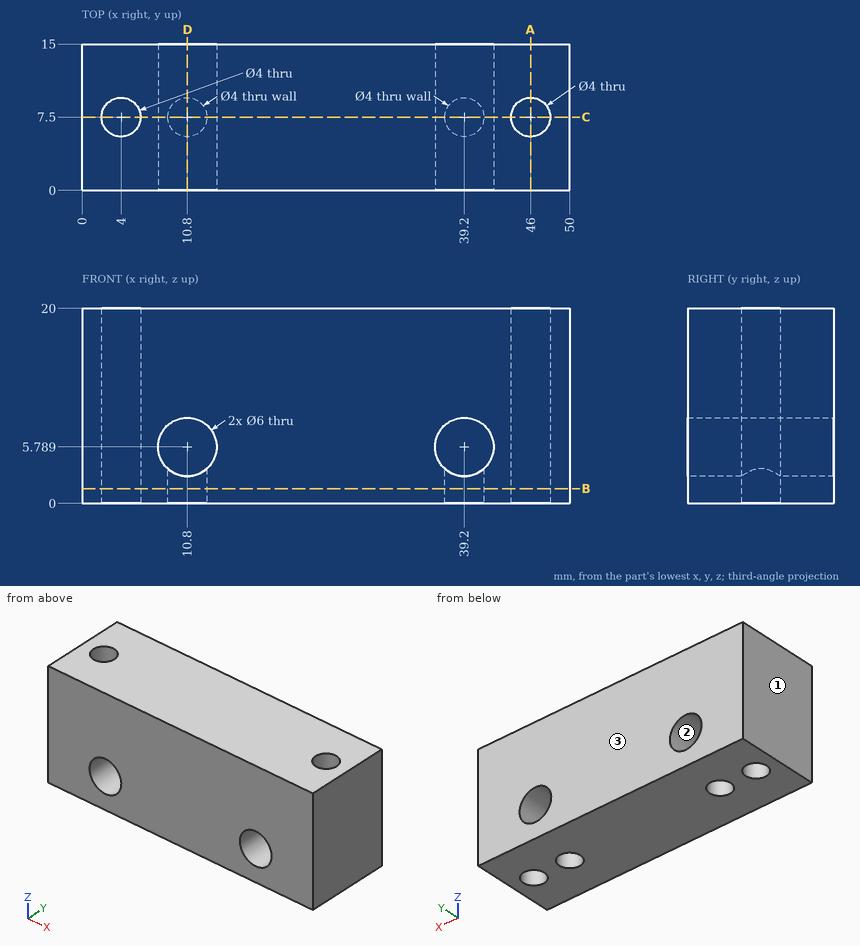
Print and shaded views of the part. All mm, measured from the part's lowest x, y and z. Round coordinates to 2 decimals unless told otherwise and drop trailing zeros. Write each loop counter-clockwise with the first axis right and the second up, starting at its lowest first coordinate (ties: lowest second). Pieces come first, ordered by that corner, then holes.
Item 1: Cut at A-A, the plane x = 46. Give the cut face in (y, z).
Results:
outline: (0, 0) - (5.5, 0) - (5.5, 20) - (0, 20) - close; (9.5, 0) - (15, 0) - (15, 20) - (9.5, 20) - close
Item 2: Two-plate mould, pull along X, no slides. Class the marked faces 1, 2 and 3: +X half, -X half, draft (parallel to the pull), parting line (faces both ways), or undercut.
Results:
face 1: -X half
face 2: undercut
face 3: draft
Item 3: Cut at D-D, the plane x = 10.8. Give the cut face in (y, z), plus the area to 3 significant figures.
Results:
outline: (0, 0) - (5.5, 0) - (5.5, 2.79) - (0, 2.79) - close; (0, 8.79) - (15, 8.79) - (15, 20) - (0, 20) - close; (9.5, 0) - (15, 0) - (15, 2.79) - (9.5, 2.79) - close
area: 199 mm2
Item 4: Cut at C-C, the plane y = 7.5. Give the cut face in (x, z), plus the area to 3 significant figures.
Results:
outline: (0, 0) - (2, 0) - (2, 20) - (0, 20) - close; (6, 0) - (8.8, 0) - (8.8, 3.55) arc R3 cw (long way) to (12.8, 3.55) - (12.8, 0) - (37.2, 0) - (37.2, 3.55) arc R3 cw (long way) to (41.2, 3.55) - (41.2, 0) - (44, 0) - (44, 20) - (6, 20) - close; (48, 0) - (50, 0) - (50, 20) - (48, 20) - close
area: 759 mm2
Item 5: Probe L1, parallel to X at y = 13.75, z = 7.25; L2, parallel to X at y = 6, z = 15; L3, parallel to Z at x = 39.2, y = 10.75. List the from-to ranges inside material, lowest first.
Results:
L1: x = 0 to 8.18, 13.42 to 36.58, 41.82 to 50
L2: x = 0 to 2.68, 5.32 to 44.68, 47.32 to 50
L3: z = 0 to 2.79, 8.79 to 20
Item 6: Cut at B-B, the plane z = 1.5. Give the cut face in (x, y).
Results:
outline: (0, 0) - (50, 0) - (50, 15) - (0, 15) - close; hole circle Ø4 at (4, 7.5); hole circle Ø4 at (10.8, 7.5); hole circle Ø4 at (39.2, 7.5); hole circle Ø4 at (46, 7.5)
